Design review of the part built by this model. Coordinates are the model's own, in mm. Coordinates: 2 decimals unless noted, no trailing zeros. Order: outer loops, then holes, each group sorted by start corner. A loop starts at its lowest first (then second) coordinate and runs counter-clockwise, first axis right, second up. Notation, with made-up numbers: M 43.25,6 L 89.25,6 A20 cw 89.25,45 Z; hole C 64,17.25 d9. An arc over 180 degrees is marked long. Use CSV: the item, a comma, the result in double quotes.
```python
from build123d import *

# Parameters (mm, degrees)
SKETCH1_R           = 5
BOSS_EXTRUDE1_DEPTH = 2


with BuildPart() as part:
    # Sketch1 → Boss-Extrude1 (new body)
    with BuildSketch(Plane.XY):
        with BuildLine():
            Line((0, 12.7), (35, 12.7))
            ThreePointArc((35, 12.7), (42.071067812, 9.771067812), (45, 2.7))
            Line((45, 2.7), (45, -2.7))
            ThreePointArc((45, -2.7), (42.071067812, -9.771067812), (35, -12.7))
            Line((35, -12.7), (0, -12.7))
            ThreePointArc((0, -12.7), (12.7, 0), (0, 12.7))
        make_face()
        with Locations((32, 0)):
            Circle(SKETCH1_R, mode=Mode.SUBTRACT)
    extrude(amount=BOSS_EXTRUDE1_DEPTH)


solid = part.part
```
(1) Add section C-C on x = 29.5. State the section outline as (y, z) points, and give its area (3 significant figures).
The answers:
outline,"M -12.7,0 L -4.33,0 L -4.33,2 L -12.7,2 Z; M 4.33,0 L 12.7,0 L 12.7,2 L 4.33,2 Z"
area,"33.5 mm2"
(2) Add section D-D on y = -10.75. State the section outline as (x, z) points, and give its area (3 significant figures).
The answers:
outline,"M 6.76,0 L 40.93,0 L 40.93,2 L 6.76,2 Z"
area,"68.3 mm2"
(3) Add section A-A on y = 0. State the section outline as (x, z) points, and give its area (3 significant figures).
The answers:
outline,"M 12.7,0 L 27,0 L 27,2 L 12.7,2 Z; M 37,0 L 45,0 L 45,2 L 37,2 Z"
area,"44.6 mm2"
(4) The part is to be moulded in two halves that separate along Y. For faces 1 (the face through (41.99, 9.85, 0.99)), 2 (the face through (12.697, -0.279, 0.986)), 3 (the face through (18, -12.7, 1)), say which applies: pulls with the +Y half, pulls with the -Y half, needs draft (parallel to the pull), parting line crosses it, or undercut.
The answers:
face 1,"pulls with the +Y half"
face 2,"undercut"
face 3,"pulls with the -Y half"
(5) Wall thickness on probe 1 along Y at (x, z) = (32, 0.85); probe 2 along Y at (x, z) = (10, 1.4); probe 3 along X at (y, z) = (-3.25, 1.95): over which ranges is each line inside the solid? List them lowest first.
The answers:
probe 1,"y = -12.7 to -5, 5 to 12.7"
probe 2,"y = -12.7 to -7.83, 7.83 to 12.7"
probe 3,"x = 12.28 to 28.2, 35.8 to 44.98"
(6) Add section B-B on z = 0.4. State the section outline as (x, y) points, and give its area (3 significant figures).
The answers:
outline,"M 0,-12.7 L 35,-12.7 A10 ccw 45,-2.7 L 45,2.7 A10 ccw 35,12.7 L 0,12.7 A12.7 cw Z; hole C 32,0 d10"
area,"768 mm2"
